Check sheet for the modelled part. Datum: model origin and axes. Units: mm. Face numbers are marked on the shaded views. A direction names the side the tool comes from. Round coordinates to 2 decimals unless told otherwise and drop trailing zeros. Write each loop counter-clockwise with the first axis right and the second up, starting at its lowest first coordinate (ties: lowest second). Pieces come first, ordered by that corner, then holes. Notation, with made-up numbers: (-35.75, 33) -> (-30.75, 33) arc R20 ccw to (-30.75, 49) -> close; hole circle Ø7 at (-40, 56). An arc over 180 degrees is marked (long way). One line per item, written item: value.
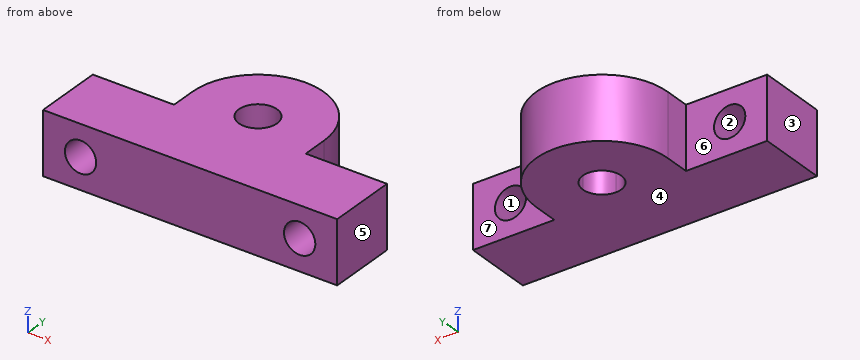
from build123d import *

# Parameters (mm, degrees)
SKETCH1_W           = 47
SKETCH1_H           = 11
BOSS_EXTRUDE1_DEPTH = 10
CUT_EXTRUDE1_REACH  = 29.807
SKETCH3_R           = 2.5
BOSS_EXTRUDE3_DEPTH = 10


with BuildPart() as part:
    # Sketch1 → Boss-Extrude1 (new body)
    with BuildSketch(Plane.XY):
        Rectangle(SKETCH1_W, SKETCH1_H)
    extrude(amount=BOSS_EXTRUDE1_DEPTH)

    # Sketch3 → Cut-Extrude1 (cut, up to next)
    with BuildSketch(Plane.XZ.offset(5.5), mode=Mode.PRIVATE) as cut_extrude1_sk1:
        with BuildLine():
            ThreePointArc((-20, 5), (-17.5, 2.5), (-15, 5))
            Line((-15, 5), (-17.5, 5))
            Line((-17.5, 5), (-20, 5))
        make_face()
    cut_extrude1_tool1 = extrude(cut_extrude1_sk1.sketch, amount=-CUT_EXTRUDE1_REACH, mode=Mode.PRIVATE) & part.part
    # Sketch3 → Cut-Extrude1 (cut, up to next)
    with BuildSketch(Plane.XZ.offset(5.5), mode=Mode.PRIVATE) as cut_extrude1_sk2:
        with BuildLine():
            Line((-17.5, 5), (-15, 5))
            ThreePointArc((-15, 5), (-17.5, 7.5), (-20, 5))
            Line((-20, 5), (-17.5, 5))
        make_face()
    cut_extrude1_tool2 = extrude(cut_extrude1_sk2.sketch, amount=-CUT_EXTRUDE1_REACH, mode=Mode.PRIVATE) & part.part
    # Sketch3 → Cut-Extrude1 (cut, up to next)
    with BuildSketch(Plane.XZ.offset(5.5), mode=Mode.PRIVATE) as cut_extrude1_sk3:
        with BuildLine():
            ThreePointArc((-20, 5), (-17.5, 2.5), (-15, 5))
            Line((-15, 5), (-17.5, 5))
            Line((-17.5, 5), (-20, 5))
        make_face()
    cut_extrude1_tool3 = extrude(cut_extrude1_sk3.sketch, amount=-CUT_EXTRUDE1_REACH, mode=Mode.PRIVATE) & part.part
    # Sketch3 → Cut-Extrude1 (cut, up to next)
    with BuildSketch(Plane.XZ.offset(5.5), mode=Mode.PRIVATE) as cut_extrude1_sk4:
        with BuildLine():
            Line((-17.5, 5), (-15, 5))
            ThreePointArc((-15, 5), (-17.5, 7.5), (-20, 5))
            Line((-20, 5), (-17.5, 5))
        make_face()
    cut_extrude1_tool4 = extrude(cut_extrude1_sk4.sketch, amount=-CUT_EXTRUDE1_REACH, mode=Mode.PRIVATE) & part.part
    # Sketch3 → Cut-Extrude1 (cut, up to next)
    with BuildSketch(Plane.XZ.offset(5.5), mode=Mode.PRIVATE) as cut_extrude1_sk5:
        with Locations(Location((17.5, 5, 0), (0, 0, 270))):
            Circle(SKETCH3_R)
    cut_extrude1_tool5 = extrude(cut_extrude1_sk5.sketch, amount=-CUT_EXTRUDE1_REACH, mode=Mode.PRIVATE) & part.part
    add(cut_extrude1_tool1.solids().sort_by_distance((-17.5, -5.5, 3.938967))[0], mode=Mode.SUBTRACT)
    add(cut_extrude1_tool2.solids().sort_by_distance((-17.5, -5.5, 6.061033))[0], mode=Mode.SUBTRACT)
    add(cut_extrude1_tool3.solids().sort_by_distance((-17.5, -5.5, 3.938967))[0], mode=Mode.SUBTRACT)
    add(cut_extrude1_tool4.solids().sort_by_distance((-17.5, -5.5, 6.061033))[0], mode=Mode.SUBTRACT)
    add(cut_extrude1_tool5.solids().sort_by_distance((17.5, -5.5, 5))[0], mode=Mode.SUBTRACT)

    # Sketch4 → Boss-Extrude3 (add)
    with BuildSketch(Plane.XY.offset(10)):
        with BuildLine():
            Line((-10.517377717, 5.5), (0, 5.5))
            Line((0, 5.5), (10.517377717, 5.5))
            Line((10.517377717, 5.5), (10.517377717, 9.5))
            ThreePointArc((10.517377717, 9.5), (0, 20.017377717), (-10.517377717, 9.5))
            Line((-10.517377717, 9.5), (-10.517377717, 5.5))
        make_face()
        with BuildLine():
            ThreePointArc((3.05, 9.5), (2.156675683, 7.343324317), (0, 6.45))
            ThreePointArc((0, 6.45), (-2.156675683, 11.656675683), (3.05, 9.5))
        make_face(mode=Mode.SUBTRACT)
    extrude(amount=-BOSS_EXTRUDE3_DEPTH)


solid = part.part
Item 1: Tool access check on the marked faces 5, 6 and 7. Record the directions out of +Z, -Z, +X, -X, +Y, -Y that give a thin tool (end or side, any length) a straight path to the whole face; none if there is none.
Result set:
face 5: +Z, -Z, +X, +Y, -Y
face 6: +Z, -Z, -X, +Y
face 7: +Z, -Z, +X, +Y
Item 2: Release check for a two-part mould opening along Z. For the marked faces 1, 2, 3 and 4 record: pulls with the +Z half, pulls with the -Z half, needs draft (parallel to the pull), parting line crosses it, or undercut.
Result set:
face 1: undercut
face 2: undercut
face 3: needs draft
face 4: pulls with the -Z half
Item 3: Sectioned sample at C-C (y = 11.25). Enter the section's corners in (x, z), then the cut area to 3 significant figures.
Result set:
outline: (-10.37, 0) -> (-2.5, 0) -> (-2.5, 10) -> (-10.37, 10) -> close; (2.5, 0) -> (10.37, 0) -> (10.37, 10) -> (2.5, 10) -> close
area: 157 mm^2
Item 4: Depth check by flat-ended pin: pin 1 (8 mm diameter, centred on x = 0, y = 9.5, fed in from -Z); pin 2 (1 mm diameter, centred on y = 6.5, z = 6.5, fed in from -X); pin 3 (3 mm diameter, centred on x = -18, z = 7, fed in from +Y); pin 4 (2 mm diameter, centred on y = 7.5, z = 4.5, fed in from +X). Enter the tip coordinate at first touch or a pass-through.
Result set:
pin 1: z = 0
pin 2: x = -10.52
pin 3: y = 5.5
pin 4: x = 10.52
Item 5: Sectioned sample at D-D (z = 1). Enter the section's corners in (x, y), then the cut area to 3 significant figures.
Result set:
outline: (-23.5, -5.5) -> (23.5, -5.5) -> (23.5, 5.5) -> (10.52, 5.5) -> (10.52, 9.5) arc R10.52 ccw to (-10.52, 9.5) -> (-10.52, 5.5) -> (-23.5, 5.5) -> close; hole circle Ø6.1 at (0, 9.5)
area: 746 mm^2
Item 6: Sectioned sample at B-B (x = -17.5). Enter the section's corners in (y, z).
Result set:
outline: (-5.5, 0) -> (5.5, 0) -> (5.5, 2.5) -> (-5.5, 2.5) -> close; (-5.5, 7.5) -> (5.5, 7.5) -> (5.5, 10) -> (-5.5, 10) -> close
Item 7: Sectioned sample at A-A (z = 5). Enter the section's corners in (x, y).
Result set:
outline: (-23.5, -5.5) -> (-20, -5.5) -> (-20, 5.5) -> (-23.5, 5.5) -> close; (-15, -5.5) -> (15, -5.5) -> (15, 5.5) -> (10.52, 5.5) -> (10.52, 9.5) arc R10.52 ccw to (-10.52, 9.5) -> (-10.52, 5.5) -> (-15, 5.5) -> close; (20, -5.5) -> (23.5, -5.5) -> (23.5, 5.5) -> (20, 5.5) -> close; hole circle Ø6.1 at (0, 9.5)
Item 8: Material ranges on line 1 along X through (y, z) = (-1, 5); line 2 along Y through (x, z) = (0, 5.25); line 3 along Z through (x, y) = (-17.5, 1), recorded low to high.
Result set:
line 1: -23.5 to -20, -15 to 15, 20 to 23.5
line 2: -5.5 to 6.45, 12.55 to 20.02
line 3: 0 to 2.5, 7.5 to 10
